Work out the finished part from the listing and answer in its coordinate system (mm). A direction names the side the tool comes from. Round coordinates to 2 decimals unless told otherwise and drop trailing zeros. Order: outer loops, then holes, each group sorted by start corner. A loop starts at its lowest first (then second) coordinate and runs counter-clockwise, first axis right, second up. Notation, with made-up numbers: (33.5, 79.5) - (38.5, 79.5) arc R8 cw to (38.5, 89.5) - close; hole circle Ø8 at (8.25, -40). An arc over 180 degrees is marked (long way). Use one line per item in the form item = value. Start each with the question number.
Q1. Find the intervals of material crossed by line 1 (Z direction, x = -10, y = -5); line 2 (X direction, y = 5, z = 27); line 3 (X direction, y = 6, z = 14.5), in increasing order. Write a range as [from, to].
Q2. The part is cut by section A-A on z = 25. Determine the outline of the cut face in (x, y).
Q3. Given P1, Ø6, axis at x = 6.5, y = -6.5, coming from the +Z side; P2, Ø0.5, axis at x = -16, z = 12.5, coming from the -Y side; P3, Ø2, axis at y = 9, z = 25.5, coming from the -X side, each flat-ended and moving along its own axis, determine where each tip first touches the part or whether it passes through.
Q4. Which of the six approach directions +Z, -Z, +X, -X, +Y, -Y give full straight-line access (tool end or side, diameter ignored) to faces 1 (the flat face through (17.52, 5.79, 15.38)), 2 (the cylindrical face through (2.28, 15.08, 13.08)), 3 (the flat face through (-16, 0, 16))?
Q5. For a pull along X with two mould halves and no side action, classify faces 4 (the cylindrical face through (3.176, 16.698, 20.935)), 5 (the flat face through (-14.526, 11.197, 15.382)), 6 (the flat face through (3.22, 16.95, 15.38)) as +X half, -X half, draft (parallel to the pull), parting line (faces both ways), or undercut.
Q6. The part is cut by section B-B on y = 12.5. Determine the outline of the cut face in (x, z).
from build123d import *

# Parameters (mm, degrees)
SKETCH_R         = 16.25
PAD_DEPTH        = 1.2
SKETCH001_W      = 1
SKETCH001_H      = 30
REVOLUTION_ANGLE = -200
PAD001_DEPTH     = 31.2
PAD002_DEPTH     = 10
HOLE_D           = 3.5
HOLE_DEPTH       = 5.85
HOLE_CSINK_D     = 7
HOLE_CSINK_ANGLE = 80
POCKET_DEPTH     = 10


with BuildPart() as part:
    # Sketch → Pad (new body)
    with BuildSketch(Plane.XY):
        Circle(SKETCH_R)
    extrude(amount=PAD_DEPTH)

    # Sketch001 → Revolution (revolve)
    with BuildSketch(Plane.XZ):
        with Locations((-15.75, 16.2)):
            Rectangle(SKETCH001_W, SKETCH001_H)
    revolve(axis=Axis((0, 0, 0), (0, 0, 1)), revolution_arc=REVOLUTION_ANGLE)

    # Sketch002 (on Face2 of Revolution) → Pad001 (join)
    with BuildSketch(Plane(origin=(0, 0, 0), x_dir=(1, 0, 0), z_dir=(0, 0, -1))):
        with BuildLine():
            Line((-16.0031258461, -2.8217836832), (-13.0076949217, -19.8097166265))
            Line((-13.0076949217, -19.8097166265), (18.9985570512, -14.1661508524))
            Line((18.9985570512, -14.1661508524), (16.0031261337, 2.8217820519))
            ThreePointArc((-16.0031258461, -2.8217836832), (2.8217828675, -16.0031259899), (16.0031261337, 2.8217820519))
        make_face()
    extrude(amount=-PAD001_DEPTH)

    # Sketch003 (on Face12 of Pad001) → Pad002 (join)
    with BuildSketch(Plane.XY.offset(31.2)):
        Polygon((-13.0076949217, 19.8097166265), (-13.4594399549, 17.2477432325), (18.546812018, 11.6041774583), (18.9985570512, 14.1661508524), align=None)
    extrude(amount=PAD002_DEPTH)

    # Hole
    with Locations(Plane(origin=(2.5436860315, 14.4259603454, 0), x_dir=(0.984807753, -0.1736481777, 0), z_dir=(-0.1736481777, -0.984807753, 0))):
        with Locations((0, 19.2)):
            CounterSinkHole(HOLE_D / 2, HOLE_CSINK_D / 2, depth=HOLE_DEPTH, counter_sink_angle=HOLE_CSINK_ANGLE)

    # Sketch005 (on Face22 of Hole) → Pocket (cut)
    with BuildSketch(Plane.XY.offset(41.2)):
        Polygon((-13.0076949217, 19.8097166265), (-13.4594399549, 17.2477432325), (18.546812018, 11.6041774583), (18.9985570512, 14.1661508524), align=None)
    extrude(amount=-POCKET_DEPTH, mode=Mode.SUBTRACT)


solid = part.part
Found:
q1.line_1 = [0, 1.2]
q1.line_2 = [-15.62, -14.41], [14.41, 17.38]
q1.line_3 = [-15.44, -14.02], [14.02, 17.56]
q2.outline = (-16.25, 0) - (-15.25, 0) arc R15.25 cw (long way) to (14.33, -5.22) - (15.27, -5.56) arc R16.25 ccw to (16, -2.82) - (19, 14.17) - (-13.01, 19.81) - (-16, 2.82) arc R16.25 ccw to start
q3.P1 = 1.2
q3.P2 = 0
q3.P3 = -15.09
q4.face_1 = +Z, -Z, +X, -Y
q4.face_2 = +Z
q4.face_3 = +Z, -X, -Y
q5.face_4 = undercut
q5.face_5 = -X half
q5.face_6 = +X half
q6.outline = (-14.3, 0) - (18.7, 0) - (18.7, 31.2) - (8.74, 31.2) - (8.74, 1.2) - (-8.74, 1.2) - (-8.74, 31.2) - (-14.3, 31.2) - close
